```python
from build123d import *

# Parameters (mm, degrees)
F0_R     = 38.1
F0_R_2   = 6.35
F1_DEPTH = 38.1
F2_R     = 5.08
F3_DEPTH = 47.625


with BuildPart() as f1:
    # F0 (on Right) → F1 (new body, symmetric)
    with BuildSketch(Plane.YZ):
        Circle(F0_R)
        Circle(F0_R_2, mode=Mode.SUBTRACT)
    extrude(amount=F1_DEPTH, both=True)

    # F2
    f2_edges = [f1.edges().sort_by_distance(p)[0] for p in [
        (38.1, -38.1, 0),
        (-38.1, -38.1, 0),
    ]]
    fillet(f2_edges, radius=F2_R)

    # F0 (on Right) → F3 (join, symmetric)
    with BuildSketch(Plane.YZ):
        Circle(F0_R_2)
    extrude(amount=F3_DEPTH, both=True)


solid = f1.part
```
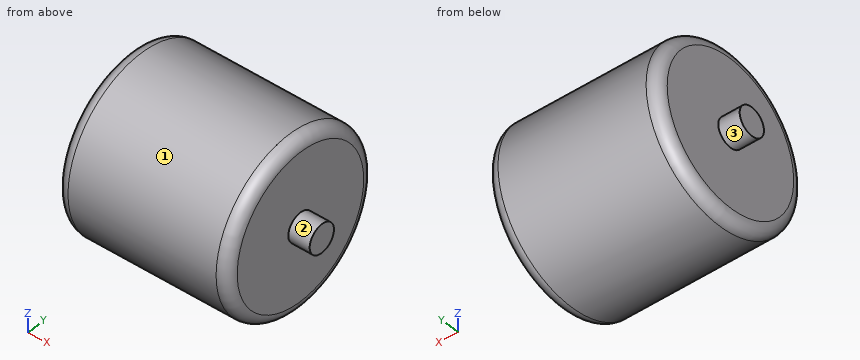
Source: CAD feature listing. Evaluate the final solid. Frame: model axes, mm. Face numbers are marked on the shaded views. A direction names the side the tool comes from. Coordinates: 2 decimals unless noted, no trailing zeros. Write each loop counter-clockwise with the first axis right and the second up, starting at its lowest first coordinate (ties: lowest second). Pieces come first, ordered by that corner, then holes. Notation, with made-up numbers: (38, 24.5) -> (94, 24.5) arc R18 ccw to (94, 47.5) -> close; hole circle Ø5 at (11, 4.5). An arc over 180 degrees is marked (long way). Return JSON: item names as keys, results as strings. Group by question number.
1) Section query A-A, the plane y = 0. Return loops of the section in (x, z) (3 decimals).
2) Section query C-C, the plane x = -41. Return loops of the section in (y, z), plus the area to 3 significant figures.
3) Section query D-D, the plane x = -10. Return loops of the section in (y, z).
4) Contact query for flat-ended pins moving along their axis: P1, Ø6, axis at x = -7, z = 7.5, coming from the +Y side; P2, Ø6, axis at x = 33, y = 22.5, coming from the -Z side; P3, Ø5, axis at x = -28, y = -15, coming from the -Z side. Output: stop coordinate, or through.
5) Set-up query: the marked faces 1, 2 and 3. Return all of +Z, -Z, +X, -X, +Y, -Y with unobstructed straight access to the full face (end or side cutting, diameter ignored); none if empty.
6) Ray query, line 1 along X through (y, z) = (19, -9.5); line 2 along Y through (x, z) = (-18, -19); line 3 along Z through (x, y) = (1, -15). Return the intervals inside material, ascending.
From the geometry:
{
 "1": {"outline": "(-47.625, -6.35) -> (-38.1, -6.35) -> (-38.1, -33.02) arc R5.08 ccw to (-33.02, -38.1) -> (33.02, -38.1) arc R5.08 ccw to (38.1, -33.02) -> (38.1, -6.35) -> (47.625, -6.35) -> (47.625, 6.35) -> (38.1, 6.35) -> (38.1, 33.02) arc R5.08 ccw to (33.02, 38.1) -> (-33.02, 38.1) arc R5.08 ccw to (-38.1, 33.02) -> (-38.1, 6.35) -> (-47.625, 6.35) -> close"},
 "2": {"outline": "circle Ø12.7 at (0, 0)", "area": "127 mm²"},
 "3": {"outline": "circle Ø76.2 at (0, 0)"},
 "4": {"P1": "y = 37.83", "P2": "z = -32.73", "P3": "z = -35.99"},
 "5": {"face 1": "+X, -X", "face 2": "+X", "face 3": "-X"},
 "6": {"line 1": "-38.1 to 38.1", "line 2": "-33.02 to 33.02", "line 3": "-35.02 to 35.02"}
}
